Build history of the part. All positions in model axes, mm. Round coordinates to 2 decimals unless told otherwise and drop trailing zeros. Loops run counter-clockwise (first coordinate to the right, second up) from the corner with the lowest first, then second, coordinate; pieces in that order, holes last.
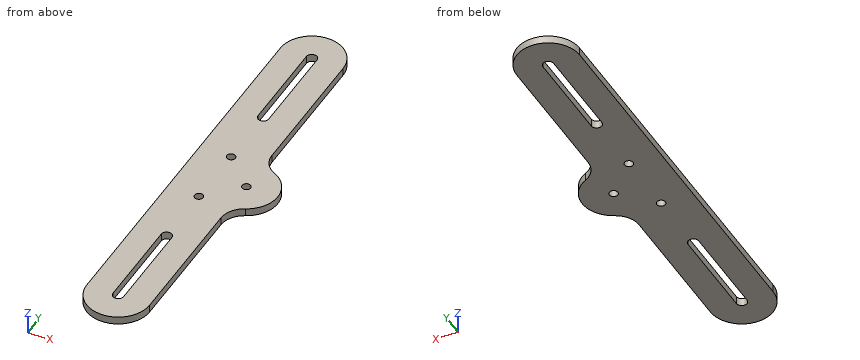
from build123d import *

# Parameters (mm, degrees)
SKETCH1_W             = 38.1
SKETCH1_H             = 177.8
BOSS_EXTRUDE1_DEPTH   = 1.5875
F_8_32_TAPPED_HOLE1_D = 3.4544
CUT_EXTRUDE1_DEPTH    = 91.973584765
SKETCH5_OUTSIDE_W     = 76.472
SKETCH5_OUTSIDE_H     = 216.172
CUT_EXTRUDE2_DEPTH    = 91.973584765


with BuildPart() as part:
    # Sketch1 → Boss-Extrude1 (new, symmetric)
    with BuildSketch(Plane.XY):
        Rectangle(SKETCH1_W, SKETCH1_H)
    extrude(amount=BOSS_EXTRUDE1_DEPTH, both=True)

    # #8-32 Tapped Hole1 (through all)
    with Locations(Plane.XY.offset(1.5875)):
        with Locations((-6.35, 12.7), (-6.35, -12.7), (6.35, 0)):
            Hole(F_8_32_TAPPED_HOLE1_D / 2)

    # Sketch4 → Cut-Extrude1 (cut, through all)
    with BuildSketch(Plane.XY.offset(1.5875)):
        with BuildLine():
            Line((-4.20116, 76.2), (-4.20116, 38.1))
            ThreePointArc((-4.20116, 38.1), (-6.35, 35.95116), (-8.49884, 38.1))
            Line((-8.49884, 38.1), (-8.49884, 76.2))
            ThreePointArc((-8.49884, 76.2), (-6.35, 78.34884), (-4.20116, 76.2))
        make_face()
        with BuildLine():
            Line((-4.20116, -38.1), (-4.20116, -76.2))
            ThreePointArc((-4.20116, -76.2), (-6.35, -78.34884), (-8.49884, -76.2))
            Line((-8.49884, -76.2), (-8.49884, -38.1))
            ThreePointArc((-8.49884, -38.1), (-6.35, -35.95116), (-4.20116, -38.1))
        make_face()
    extrude(amount=-CUT_EXTRUDE1_DEPTH, mode=Mode.SUBTRACT)

    # Sketch5 outside → Cut-Extrude2 (cut, through all)
    with BuildSketch(Plane.XY.offset(1.5875)):
        Rectangle(SKETCH5_OUTSIDE_W, SKETCH5_OUTSIDE_H)
        with BuildLine():
            Line((6.35, 76.2), (6.35, 20.080463142))
            ThreePointArc((6.35, 20.080463142), (7.824905724, 14.989136484), (11.792857143, 11.474550367))
            ThreePointArc((11.792857143, 11.474550367), (19.05, 0), (11.792857143, -11.474550367))
            ThreePointArc((11.792857143, -11.474550367), (7.824905724, -14.989136484), (6.35, -20.080463142))
            Line((6.35, -20.080463142), (6.35, -76.2))
            ThreePointArc((6.35, -76.2), (-6.35, -88.9), (-19.05, -76.2))
            Line((-19.05, -76.2), (-19.05, 76.2))
            ThreePointArc((-19.05, 76.2), (-6.35, 88.9), (6.35, 76.2))
        make_face(mode=Mode.SUBTRACT)
    extrude(amount=-CUT_EXTRUDE2_DEPTH, mode=Mode.SUBTRACT)


solid = part.part
(1) Probe line 1 (Y direction, x = -6.35, z = 0.65); line 2 (X direction, y = 41.5, z = 0.4); line 3 (X direction, y = -22, z = -0.35). List the from-to ranges inside material, lowest first.
Responses:
line 1: y = -88.9 to -78.35, -35.95 to -14.43, -10.97 to 10.97, 14.43 to 35.95, 78.35 to 88.9
line 2: x = -19.05 to -8.5, -4.2 to 6.35
line 3: x = -19.05 to 6.35
(2) Slice it at C-C on y = -29. List the corners of the cut face in (x, z), plus the area to 3 significant figures.
Responses:
outline: (-19.05, -1.59) - (6.35, -1.59) - (6.35, 1.59) - (-19.05, 1.59) - close
area: 80.6 mm2
(3) Pin check, flat tips, straight feed: P1, Ø1.5, axis at x = -3, z = 0, coming from the -Y side; P2, Ø1, axis at y = -34.5, z = 0.5, coming from the +X side. Stop position of each tip, or through.
Responses:
P1: stops at y = -88.63
P2: stops at x = 6.35
(4) Slice it at D-D on x = 14. List the corners of the cut face in (y, z).
Responses:
outline: (-10.14, -1.59) - (10.14, -1.59) - (10.14, 1.59) - (-10.14, 1.59) - close
(5) Slice it at B-B on z = -0.05. List the corners of the cut face in (x, y) (3 decimals).
Responses:
outline: (-19.05, -76.2) arc R12.7 ccw to (6.35, -76.2) - (6.35, -20.08) arc R9.525 cw to (11.793, -11.475) arc R12.7 ccw to (11.793, 11.475) arc R9.525 cw to (6.35, 20.08) - (6.35, 76.2) arc R12.7 ccw to (-19.05, 76.2) - close; hole (-8.499, -76.2) arc R2.149 ccw to (-4.201, -76.2) - (-4.201, -38.1) arc R2.149 ccw to (-8.499, -38.1) - close; hole (-8.499, 38.1) arc R2.149 ccw to (-4.201, 38.1) - (-4.201, 76.2) arc R2.149 ccw to (-8.499, 76.2) - close; hole circle Ø3.454 at (-6.35, -12.7); hole circle Ø3.454 at (-6.35, 12.7); hole circle Ø3.454 at (6.35, 0)
(6) Slice it at A-A on y = 68.5. List the corners of the cut face in (x, z).
Responses:
outline: (-19.05, -1.59) - (-8.5, -1.59) - (-8.5, 1.59) - (-19.05, 1.59) - close; (-4.2, -1.59) - (6.35, -1.59) - (6.35, 1.59) - (-4.2, 1.59) - close
